Check sheet for the modelled part. Datum: model origin and axes. Units: mm. Face numbers are marked on the shaded views. A direction names the side the tool comes from. Round coordinates to 2 decimals unless told otherwise and drop trailing zeros. Loops run counter-clockwise (first coordinate to the right, second up) from the corner with the lowest first, then second, coordinate; pieces in that order, holes last. Notation, with made-up numbers: (60, 1.5) - (67, 1.5) arc R19 ccw to (67, 37.5) - close; hole circle Ø5 at (13.5, 21.5). An arc over 180 degrees is marked (long way). Answer in a Markdown table with one row per item. Add a question column.
(1) Gauge pin test, flat ends, axial feed: pin 1 (10 mm diameter, centred on x = -17, z = -1.5, fed in from +Y); pin 2 (5 mm diameter, centred on x = -4, z = -1, fed in from +Y); pin 3 (4 mm diameter, centred on x = -5.5, y = -2, fed in from -Z); pin 4 (3.5 mm diameter, centred on x = -9.525, z = 0, fed in from +Y). Record the tip position at first contact, or that the pin passes through.
(2) Access from +Z, -Z, +X, -X, +Y, -Y to the whole of each face (thin tool, end or side, straight path). Record for the marked faces 1 and 2.
(3) Cross-section at B-B on x = -9.25. Enter the section's corners in (y, z) (3 decimals), then the cut area to 3 significant figures.
(4) Cross-section at C-C on y = 4.75. Enter the section's corners in (x, z) (3 decimals).
(5) Cross-section at D-D on z = 3. Enter the section's corners in (x, y) (1 decimal), then the cut area to 3 significant figures.
(6) Thickness scan on line 1 along X through (y, z) = (0, 3); line 2 along X through (y, z) = (-1.25, 5); line 3 along Z through (x, y) = (-8.5, 6). Record the ranges inside material, lowest first.
Autodesk Inventor part; units mm, degrees
ref_plane "Work Plane1" through (-9.525, 9.525, 0) normal (0, 1, 0) x (-1, 0, 0)
ref_plane "Work Plane2" through (0, 0, 9.525) normal (0, 0, 1) x (1, 0, 0)
ref_plane "YZ Plane" through (0, 0, 0) normal (1, 0, 0) x (0, 1, 0)
sketch "Sketch1" plane through (0, 0, 0) normal (0, 1, 0) x (-1, 0, 0)
  line L0 (0, 0) -> (19.05, 0)
  arc A0 (19.05, 0) -> (0, 0) centre (9.525, 0) ccw
  dimension "d0" = 19.05
revolve "Revolution1" add sketch "Sketch1" angle 360 about axis through (0, 0, 0) along (-1, 0, 0)
ref_plane "Work Plane1" through (-9.525, 9.525, 0) normal (0, 1, 0) x (-1, 0, 0)
ref_plane "Work Plane2" through (0, 0, 9.525) normal (0, 0, 1) x (1, 0, 0)
sketch "Sketch5" plane through (-9.525, 9.525, 0) normal (0, 1, 0) x (-1, 0, 0)
  circle A0 centre (0, 0) radius 1.3208
  point P0 (-9.525, 0)
  dimension "d19" = 2.6416
  dimension "d20" = 9.525
extrude "Extrusion1" cut sketch "Sketch5" against normal through all
sketch "Sketch6" plane through (0, 0, 9.525) normal (0, 0, 1) x (1, 0, 0)
  circle A0 centre (-9.525, 0) radius 3.7465
  point P0 (0, 0)
  dimension "d23" = 9.525
  dimension "d24" = 7.493
extrude "Extrusion2" cut sketch "Sketch6" against normal blind 12.7
properties part number "VS-008 (HANDLE BALL)" material "Steel, Carbon"
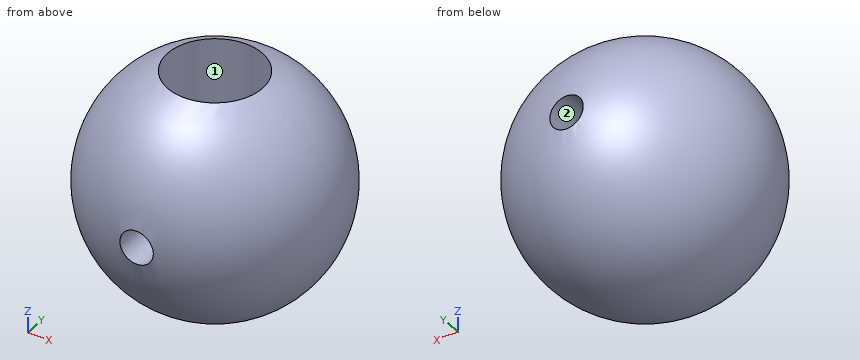
Answers:
| question | item | result |
|---|---|---|
| 1 | pin 1 | stops at y = 9.16 |
| 1 | pin 2 | stops at y = 9 |
| 1 | pin 3 | stops at z = -9.19 |
| 1 | pin 4 | stops at y = 9.43 |
| 2 | face 1 | +Z |
| 2 | face 2 | +Y, -Y |
| 3 | outline | (-9.433, -1.292) arc R9.521 ccw to (9.433, -1.292) - (3.736, -1.292) - (3.736, -3.175) - (-3.736, -3.175) - (-3.736, -1.292) - close; (-9.433, 1.292) - (-3.736, 1.292) - (-3.736, 8.757) arc R9.521 ccw to start; (3.736, 1.292) - (9.433, 1.292) arc R9.521 ccw to (3.736, 8.757) - close |
| 3 | area | 162 mm^2 |
| 4 | outline | circle Ø16.512 at (-9.525, 0); hole circle Ø2.642 at (-9.525, 0) |
| 5 | outline | circle Ø18.1 at (-9.5, 0); hole circle Ø7.5 at (-9.5, 0) |
| 5 | area | 213 mm^2 |
| 6 | line 1 | x = -18.57 to -13.27, -5.78 to -0.48 |
| 6 | line 2 | x = -17.54 to -13.06, -5.99 to -1.51 |
| 6 | line 3 | z = -7.33 to -0.83, 0.83 to 7.33 |
